Geometry check sheet. Reference: drawing and pictorial views, mm from the part's lowest x, y, z. Round coordinates to 2 decimals unless told otherwise and drop trailing zeros. Order: outer loops, then holes, each group sorted by start corner. A loop starts at its lowest first (then second) coordinate and runs counter-clockwise, first axis right, second up.
(1) Sectioned sample at D-D (y = 0.65). Record the boundary of the cut face in (x, z).
(2) Sectioned sample at C-C (z = 37.5). Record the boundary of the cut face in (x, y).
(3) Material ranges on line 1 along X through (y, z) = (3.25, 77); line 2 along X through (y, z) = (3.1, 24); line 3 along Z through (x, y) = (3.5, 2.4), recorded low to high.
(4) Sectioned sample at B-B (x = 14). Record the boundary of the cut face in (y, z).
(5) Sectioned sample at A-A (z = 24). Record the boundary of the cut face in (x, y), plus the area to 3 significant figures.
(6) Go/stop test with flat-tipped pins: pin 1 (2.5 mm diameter, centred on x = 12, z = 24, fed in from -Y); pin 2 (0.6 mm diameter, centred on y = 1.5, z = 39, fed in from +X); pin 3 (1.6 mm diameter, centred on x = 3.5, y = 0.5, fed in from -Z). Record where each tip stops, or that it passes through.
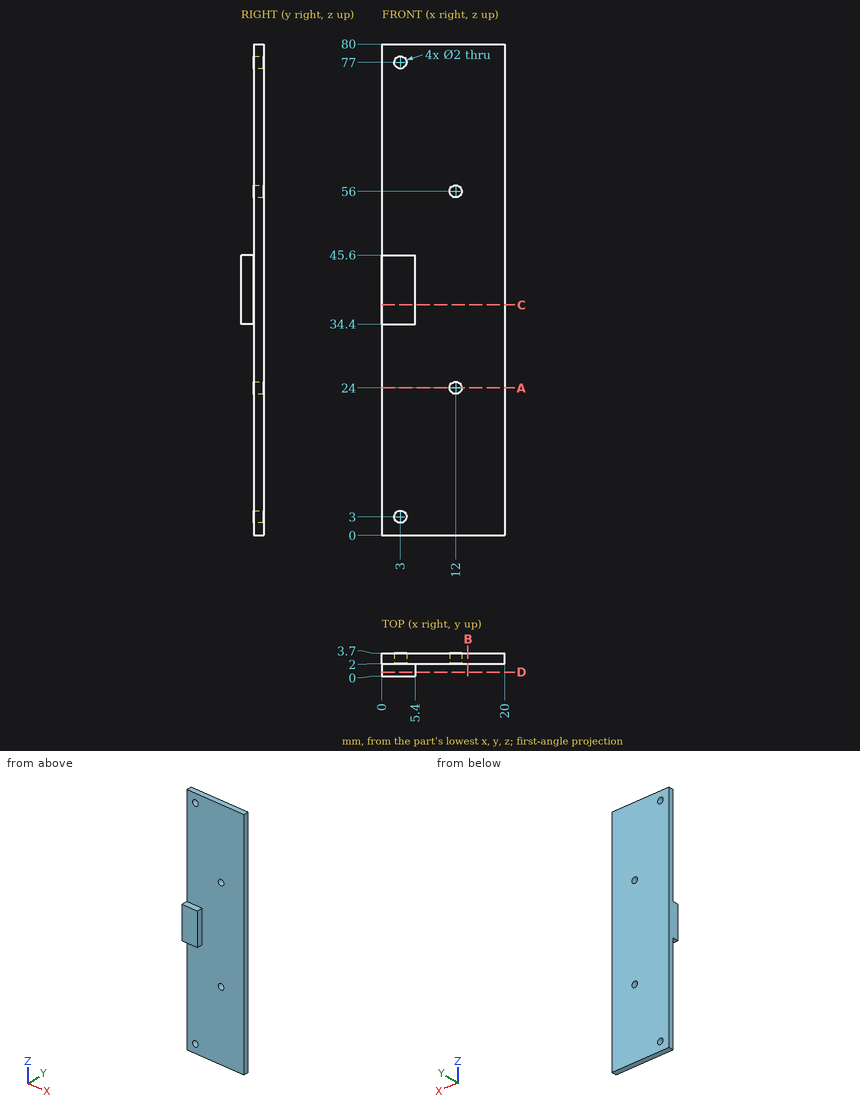
Answer below:
1. outline: (0, 34.4) - (5.4, 34.4) - (5.4, 45.6) - (0, 45.6) - close
2. outline: (0, 0) - (5.4, 0) - (5.4, 2) - (20, 2) - (20, 3.7) - (0, 3.7) - close
3. line 1: x = 0 to 2, 4 to 20
3. line 2: x = 0 to 11, 13 to 20
3. line 3: z = 0 to 2.13, 3.87 to 76.13, 77.87 to 80
4. outline: (2, 0) - (3.7, 0) - (3.7, 80) - (2, 80) - close
5. outline: (0, 2) - (11, 2) - (11, 3.7) - (0, 3.7) - close; (13, 2) - (20, 2) - (20, 3.7) - (13, 3.7) - close
5. area: 30.6 mm2
6. pin 1: stops at y = 2
6. pin 2: stops at x = 5.4
6. pin 3: stops at z = 34.4
